Geometry check sheet. Reference: the model listing, model coordinates, mm. Face numbers are marked on the shaded views. A direction names the side the tool comes from. Coordinates: 2 decimals unless noted, no trailing zeros. Write each loop counter-clockwise with the first axis right and the second up, starting at its lowest first coordinate (ties: lowest second). Pieces come first, ordered by that corner, then holes. Notation, with made-up numbers: (18, 3.25) -> (27, 3.25) arc R8 ccw to (27, 8.25) -> close; hole circle Ø7 at (6.5, 86). An arc over 180 degrees is marked (long way). Use a Markdown table: item, result.
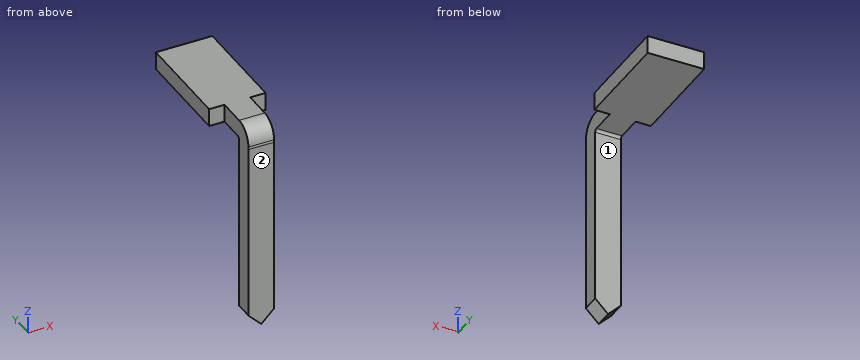
Autodesk Inventor part; units mm, degrees
ref_plane "YZ Plane" through (0, 0, 0) normal (1, 0, 0) x (0, 1, 0)
ref_plane "XZ Plane" through (0, 0, 0) normal (0, 1, 0) x (-1, 0, 0)
ref_plane "XY Plane" through (0, 0, 0) normal (0, 0, 1) x (1, 0, 0)
sketch "Sketch1" plane through (0, 0, 0) normal (0, 0, 1) x (1, 0, 0)
  line L0 (1.1, 0) -> (-1.1, 0)
  line L1 (-1.1, 0) -> (-1.1, -4)
  line L2 (-1.1, -4) -> (-0.5, -4)
  line L3 (-0.5, -4) -> (-0.5, -17)
  line L4 (-0.5, -17) -> (0, -17.5)
  line L5 (0, -17.5) -> (0.5, -17)
  line L6 (0.5, -17) -> (0.5, -4)
  line L7 (0.5, -4) -> (1.1, -4)
  line L8 (1.1, -4) -> (1.1, 0)
  line L9 (0, 0) -> (0, -17.5) construction
  dimension "d0" = 2.2
  dimension "d1" = 17.5
  dimension "d3" = 1
  dimension "d4" = 4
  dimension "d5" = -45
extrude "Extrusion1" add sketch "Sketch1" along normal blind 0.7
sketch "Sketch2" plane through (0, 0, 0.7) normal (0, 0, 1) x (1, 0, 0)
  line L0 (1.1, 0) -> (-1.1, 0)
  line L1 (-0.5, -4) -> (-0.5, -17)
  line L2 (0.5, -17) -> (0.5, -4)
  point P0 (0, 0)
  point P1 (-0.5, -5)
  point P2 (0.5, -5)
extrude "Extrusion2" [suppressed]
sketch "Sketch3" plane through (0.5, -4, 0.7) normal (1, 0, 0) x (0, 0, -1)
  line L0 (0.7, 0) -> (0.7, -13)
  line L1 (0.8, -1.1) -> (8.2, -1.1)
  line L2 (8.2, -1.1) -> (8.2, -1.8)
  line L3 (8.2, -1.8) -> (0.8, -1.8)
  arc A0 (0.7, -1) -> (0.8, -1.1) centre (0.8, -1) ccw
  line L4 (0.7, -13) -> (0.7, 0)
  arc A1 (0, -1) -> (0.8, -1.8) centre (0.8, -1) ccw
  line L5 (0, -13) -> (0, 0)
  line L6 (0, -1) -> (0.7, -1)
  line L7 (0, -1) -> (0.7, -1)
  point P0 (0.7, 4)
  dimension "d12" = 0.7
  dimension "d19" = 0.1
  dimension "d20" = 0.7
  dimension "d21" = 7.5
extrude "Extrusion5" add sketch "Sketch3" against normal blind 1
sketch "Sketch5" plane through (0.5, -5.1, -0.1) normal (0, 1, 0) x (1, 0, 0)
  line L0 (-1, 0) -> (-1, 7.4)
  line L1 (-1, 6.9) -> (-0.5, 7.4)
  line L2 (-0.5, 7.4) -> (-1, 7.4)
  line L3 (-1, 7.4) -> (-1, 6.9)
  line L4 (-0.5, 7.4) -> (0, 6.9)
  line L5 (0, 7.4) -> (-1, 7.4)
  line L6 (0, 6.9) -> (0, 7.4)
  line L7 (0, 7.4) -> (-0.5, 7.4)
  line L8 (0, 0) -> (-1, 0) construction
  line L9 (-0.5, 0) -> (-0.5, 7.4) construction
  point P0 (-0.5, -0.1)
  dimension "d25" = 90
extrude "Extrusion6" cut sketch "Sketch5" against normal blind 1
sketch "Sketch6" plane through (0.5, -17, 0.7) normal (1, 0, 0) x (0, 0, -1)
  line L0 (0.7, 0) -> (0.7, 11.2063)
  line L1 (0, -0.5) -> (0, 0)
  line L2 (0.7, 11.2063) -> (0, 11.2063)
  line L3 (0, 11.2063) -> (0, -0.5)
  line L4 (0, -0.5) -> (0.7, -0.5)
  line L5 (0.7, -0.5) -> (0.7, 11.2063)
  point P0 (0.7, 17)
extrude "Extrusion7" cut sketch "Sketch6" against normal blind 10
fillet "Fillet2" radius 0.7 1 edges at (0, -5.7937, 0.7)
properties part number "BrueckenGR_LVE2560E_Feet" material "Nickel-Copper Alloy 400"
Item 1: Depth check by flat-ended pin: P1, Ø0.5, axis at y = -5, z = -3, coming from the +X side; P2, Ø0.7, axis at x = -0.5, z = 0.5, coming from the -Y side; P3, Ø0.9, axis at y = -5.5, z = -2, coming from the -X side. Enter the tip coordinate at first touch or a pass-through.
Answer block:
| item | result |
|---|---|
| P1 | stops at x = 0.5 |
| P2 | stops at y = -5.78 |
| P3 | stops at x = -0.5 |
Item 2: Section check B-B on y = -4.2. Record the boundary of the cut face in (x, z).
Answer block:
| item | result |
|---|---|
| outline | (-0.5, 0) -> (0.5, 0) -> (0.5, 0.7) -> (-0.5, 0.7) -> close |
Item 3: Section check C-C on z = -4.5. Record the boundary of the cut face in (x, y), then the cut area to 3 significant figures.
Answer block:
| item | result |
|---|---|
| outline | (-0.5, -5.8) -> (0.5, -5.8) -> (0.5, -5.1) -> (-0.5, -5.1) -> close |
| area | 0.700 mm^2 |
Item 4: Thickness scan on L1, parallel to Y at x = 0.35, z = -4.5; L2, parallel to Z at x = 0.45, y = -4.5. Record the ranges inside material, lowest first. Write a range as [from, to].
Answer block:
| item | result |
|---|---|
| L1 | y = [-5.8, -5.1] |
| L2 | z = [0, 0.7] |
Item 5: Tool access check on the marked faces 1 and 2. Record the directions out of +Z, -Z, +X, -X, +Y, -Y that give a thin tool (end or side, any length) a straight path to the whole face; none if there is none.
Answer block:
| item | result |
|---|---|
| face 1 | -Z, +X, -X, +Y |
| face 2 | +Z, -Z, +X, -X, -Y |
